Source: three-view drawing plus pictorial views. Frame: mm from the lowest corner of the part. A direction names the side the tool comes from. Give positions to 0.01 mm unless a question says otherwise; leave off trailing zeros. Write each loop counter-clockwise with the first axis right and the second up, starting at its lowest first coordinate (ties: lowest second). Pieces come first, ordered by that corner, then holes. Notation, with made-up numbers: (-18, 76) -> (18, 76) arc R14 cw to (18, 90) -> close; hole circle Ø6 at (-6.5, 40.25). An arc over 180 degrees is marked (long way). Write item = value, one per line.
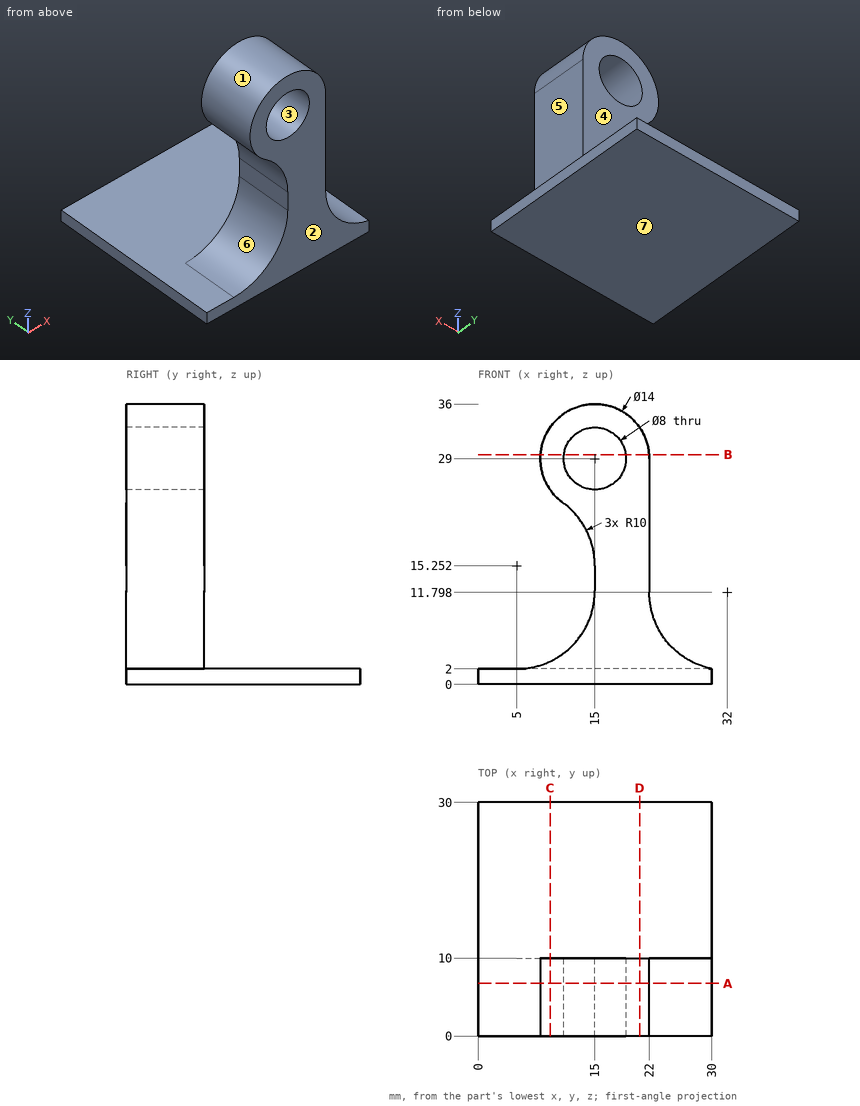
1) Draft query along X for the marked faces 1, 2 and 3. Return one class per face: pulls with the +X half, pulls with the -X half, needs draft (parallel to the pull), parting line crosses it, or undercut.
Computed:
face_1 = parting line crosses it
face_2 = needs draft
face_3 = undercut
2) Cut plane C-C (x = 9.25). Return the cut outline in (y, z).
Computed:
outline = (0, 0) -> (30, 0) -> (30, 2) -> (10, 2) -> (10, 2.95) -> (0, 2.95) -> close; (0, 25.01) -> (10, 25.01) -> (10, 32.99) -> (0, 32.99) -> close
3) Cut plane A-A (y = 6.75). Return the cut outline in (x, z).
Computed:
outline = (0, 0) -> (30, 0) -> (30, 2) arc R10 cw to (22, 11.8) -> (22, 29) arc R7 ccw (long way) to (10.88, 23.34) arc R10 cw to (15, 15.25) -> (15, 12) arc R10 cw to (5, 2) -> (0, 2) -> close; hole circle Ø8 at (15, 29)
4) Contact query for flat-ended pins moving along their axis: pin 1 (2.5 mm diameter, centred on y = 5.5, z = 14, fed in from -X); pin 2 (12.5 mm diameter, centred on x = 19.5, z = 24.5, fed in from +Y); pin 3 (2 mm diameter, centred on x = 16.5, z = 31, fed in from -Y); pin 4 (2 mm diameter, centred on y = 10.5, z = 24.5, fed in from +X). Output: stop coordinate, or through.
Computed:
pin_1 = 15
pin_2 = 10
pin_3 = through
pin_4 = 22
5) Cut plane D-D (x = 20.75). Return the cut outline in (y, z).
Computed:
outline = (0, 0) -> (30, 0) -> (30, 2) -> (10, 2) -> (10, 32.99) -> (0, 32.99) -> close
6) Cut plane B-B (z = 29.5). Return the cut outline in (x, y).
Computed:
outline = (8.02, 0) -> (11.03, 0) -> (11.03, 10) -> (8.02, 10) -> close; (18.97, 0) -> (21.98, 0) -> (21.98, 10) -> (18.97, 10) -> close
7) Material intervals for L1, parallel to Z at x = 11.5, y = 15.5; L2, parallel to X at y = 5, z = 15; L3, parallel to X at y = 7, z = 32 (1 decimal), sorted ascending.
Computed:
L1 = 0 to 2
L2 = 15 to 22
L3 = 8.7 to 12.4, 17.6 to 21.3
8) Access query for the marked faces 4, 5, 6 and 7. Directions: +Z, -Z, +X, -X, +Y, -Y. A direction counts if a zero-diameter tool reaches every point of the face in a straight line with its end or side. Return the directions, or none.
Computed:
face_4 = +Z, +X, -X, +Y
face_5 = +Z, +X, +Y, -Y
face_6 = -X, +Y, -Y
face_7 = -Z, +X, -X, +Y, -Y
